```python
from build123d import *

# Parameters (mm, degrees)
SKETCH1_W           = 101.6
SKETCH1_H           = 247.65
BOSS_EXTRUDE1_DEPTH = 152.4
SKETCH2_R           = 15.08125
SKETCH2_R_2         = 9.525
CUT_EXTRUDE1_DEPTH  = 203.827588422
CUT_EXTRUDE2_DEPTH  = 222.090367554
SKETCH33_R          = 2.5796875
CUT_EXTRUDE33_DEPTH = 25.4
SKETCH53_R          = 31.75
CUT_EXTRUDE37_DEPTH = 24.13
SKETCH54_R          = 19.05
CUT_EXTRUDE38_DEPTH = 38.1
SKETCH4_R           = 19.05
CUT_EXTRUDE40_DEPTH = 12.7
SKETCH55_R          = 1.7859375
CUT_EXTRUDE41_DEPTH = 25.4
SKETCH56_R          = 14.2494
CUT_EXTRUDE42_DEPTH = 12.7
CUT_EXTRUDE43_START = -12.7
SKETCH57_R          = 14.2494
CUT_EXTRUDE43_DEPTH = 12.7
SKETCH58_R          = 25.4
CUT_EXTRUDE44_DEPTH = 50.8
CUT_EXTRUDE45_DEPTH = 127
FILLET2_R           = 0.00254
CUT_EXTRUDE46_START = -12.7
SKETCH60_R          = 19.05
CUT_EXTRUDE46_DEPTH = 12.7
SKETCH61_R          = 9.525
CUT_EXTRUDE47_DEPTH = 222.090367554
SKETCH62_R          = 2.0193
CUT_EXTRUDE48_DEPTH = 25.4
SKETCH63_R          = 3.175
CUT_EXTRUDE49_DEPTH = 12.7


with BuildPart() as part:
    # Sketch1 → Boss-Extrude1 (new body)
    with BuildSketch(Plane.XY):
        Rectangle(SKETCH1_W, SKETCH1_H)
    extrude(amount=BOSS_EXTRUDE1_DEPTH)

    # Sketch2 → Cut-Extrude1 (cut, through all)
    with BuildSketch(Plane(origin=(0, 0, 0), x_dir=(-1, 0, 0), z_dir=(0, 0, -1))):
        with Locations((0, -60.579)):
            Circle(SKETCH2_R)
        with Locations((0, 53.721)):
            Circle(SKETCH2_R_2)
    extrude(amount=-CUT_EXTRUDE1_DEPTH, mode=Mode.SUBTRACT)

    # Sketch3 → Cut-Extrude2 (cut, through all)
    with BuildSketch(Plane.ZY.offset(50.8)):
        Polygon((152.4, -60.325), (88.9, -123.825), (152.4, -123.825), align=None)
    extrude(amount=-CUT_EXTRUDE2_DEPTH, mode=Mode.SUBTRACT)

    # Sketch33 → Cut-Extrude33 (cut)
    with BuildSketch(Plane(origin=(0, 0, 0), x_dir=(-1, 0, 0), z_dir=(0, 0, -1))):
        with Locations((-40.005, 102.9335)):
            Circle(SKETCH33_R)
        with Locations((40.005, 102.9335)):
            Circle(SKETCH33_R)
        with Locations((40.005, 4.5085)):
            Circle(SKETCH33_R)
        with Locations((-40.005, 4.5085)):
            Circle(SKETCH33_R)
    extrude(amount=-CUT_EXTRUDE33_DEPTH, mode=Mode.SUBTRACT)

    # Sketch53 → Cut-Extrude37 (cut)
    with BuildSketch(Plane(origin=(0, 0, 0), x_dir=(-1, 0, 0), z_dir=(0, 0, -1))):
        with Locations((0, -60.579)):
            Circle(SKETCH53_R)
    extrude(amount=-CUT_EXTRUDE37_DEPTH, mode=Mode.SUBTRACT)

    # Sketch54 → Cut-Extrude38 (cut)
    with BuildSketch(Plane(origin=(0, 0, 0), x_dir=(-1, 0, 0), z_dir=(0, 0, -1))):
        with Locations((0, 53.721)):
            Circle(SKETCH54_R)
    extrude(amount=-CUT_EXTRUDE38_DEPTH, mode=Mode.SUBTRACT)

    # Sketch4 → Cut-Extrude40 (cut)
    with BuildSketch(Plane(origin=(50.8, 0, 0), x_dir=(0, 0, -1), z_dir=(1, 0, 0))):
        with Locations((-76.2, 28.575)):
            Circle(SKETCH4_R)
    extrude(amount=-CUT_EXTRUDE40_DEPTH, mode=Mode.SUBTRACT)

    # Sketch55 → Cut-Extrude41 (cut)
    with BuildSketch(Plane.ZY.offset(50.8)):
        with Locations((52.3875, 28.575)):
            Circle(SKETCH55_R)
        with Locations((64.29375, 49.197229928)):
            Circle(SKETCH55_R)
        with Locations((88.10625, 49.197229928)):
            Circle(SKETCH55_R)
        with Locations((100.0125, 28.575)):
            Circle(SKETCH55_R)
        with Locations((88.10625, 7.952770072)):
            Circle(SKETCH55_R)
        with Locations((64.29375, 7.952770072)):
            Circle(SKETCH55_R)
    cut_extrude41 = extrude(amount=-CUT_EXTRUDE41_DEPTH, mode=Mode.SUBTRACT)

    # Sketch56 → Cut-Extrude42 (cut)
    with BuildSketch(Plane.XY.offset(152.4)):
        with Locations((0, 53.721)):
            Circle(SKETCH56_R)
    extrude(amount=-CUT_EXTRUDE42_DEPTH, mode=Mode.SUBTRACT)

    # Sketch57 → Cut-Extrude43 (cut)
    with BuildSketch(Plane(origin=(0, 0, 38.1), x_dir=(-1, 0, 0), z_dir=(0, 0, -1)).offset(CUT_EXTRUDE43_START)):
        with Locations(Location((0, 53.721, 0), (0, 0, 180))):
            Circle(SKETCH57_R)
    extrude(amount=CUT_EXTRUDE43_DEPTH, mode=Mode.SUBTRACT)

    # Sketch58 → Cut-Extrude44 (cut)
    with BuildSketch(Plane.XY.offset(152.4)):
        with Locations((0, -60.579)):
            Circle(SKETCH58_R)
    extrude(amount=-CUT_EXTRUDE44_DEPTH, mode=Mode.SUBTRACT)

    # Sketch59 → Cut-Extrude45 (cut)
    with BuildSketch(Plane.XY.offset(152.4)):
        with BuildLine():
            ThreePointArc((-17.734642857, -13.34047826), (20.0025, -4.0894), (-17.734642857, 5.16167826))
            ThreePointArc((-17.734642857, 5.16167826), (-29.5275, -4.0894), (-17.734642857, -13.34047826))
        make_face()
    extrude(amount=-CUT_EXTRUDE45_DEPTH, mode=Mode.SUBTRACT)

    # Fillet2
    fillet2_edges = [part.edges().sort_by_distance(p)[0] for p in [
        (50.8, -123.825, 44.45),
        (-50.8, -123.825, 44.45),
        (-50.8, 123.825, 76.2),
        (50.8, 123.825, 76.2),
    ]]
    fillet(fillet2_edges, radius=FILLET2_R)

    # Sketch60 → Cut-Extrude46 (cut)
    with BuildSketch(Plane.ZY.offset(50.8).offset(CUT_EXTRUDE46_START)):
        with Locations(Location((76.2, 28.575, 0), (0, 0, 180))):
            Circle(SKETCH60_R)
    extrude(amount=CUT_EXTRUDE46_DEPTH, mode=Mode.SUBTRACT)

    # Sketch61 → Cut-Extrude47 (cut, through all)
    with BuildSketch(Plane(origin=(50.8, 0, 0), x_dir=(0, 0, -1), z_dir=(1, 0, 0))):
        with Locations((-76.2, 28.575)):
            Circle(SKETCH61_R)
    extrude(amount=-CUT_EXTRUDE47_DEPTH, mode=Mode.SUBTRACT)

    # Sketch62 → Cut-Extrude48 (cut)
    with BuildSketch(Plane.XY.offset(152.4)):
        with Locations((-22.225, 18.1356)):
            Circle(SKETCH62_R)
        with Locations((22.225, 18.1356)):
            Circle(SKETCH62_R)
        with Locations((22.225, -26.3144)):
            Circle(SKETCH62_R)
        with Locations((-22.225, -26.3144)):
            Circle(SKETCH62_R)
    extrude(amount=-CUT_EXTRUDE48_DEPTH, mode=Mode.SUBTRACT)

    # Sketch63 → Cut-Extrude49 (cut)
    with BuildSketch(Plane(origin=(50.8, 0, 0), x_dir=(0, 0, -1), z_dir=(1, 0, 0))):
        with Locations((-50.8, 66.675)):
            Circle(SKETCH63_R)
        with Locations((-12.7, 66.675)):
            Circle(SKETCH63_R)
        with Locations((-12.7, 92.075)):
            Circle(SKETCH63_R)
        with Locations((-50.8, 92.075)):
            Circle(SKETCH63_R)
    extrude(amount=-CUT_EXTRUDE49_DEPTH, mode=Mode.SUBTRACT)

    # Mirror2: Cut-Extrude41 across plane
    add(cut_extrude41.mirror(Plane(origin=(0, 0, 0), x_dir=(0, 0, 1), z_dir=(1, 0, 0))), mode=Mode.SUBTRACT)


solid = part.part
```
Part model, mm, in its own coordinate system. A direction names the side the tool comes from. Round coordinates to 2 decimals unless told otherwise and drop trailing zeros. Order: outer loops, then holes, each group sorted by start corner. A loop starts at its lowest first (then second) coordinate and runs counter-clockwise, first axis right, second up. Notation, with made-up numbers: M 7.25,27.5 L 66.25,27.5 A20 ccw 66.25,54.5 Z; hole C -3,-15 d7. An arc over 180 degrees is marked long. Answer in a Markdown table with one row per item. Add a question column.
Q1. Mould opens along Z. For faces 1 (the face through (-1, 33, 152.4)), 2 (the face through (1.24, 63.165, 94.628)), 3 (the face through (0.533, 28.994, 85.716)) say: +Z half, -Z half, draft (parallel to the pull), parting line (faces both ways), or undercut.
Q2. Pin check, flat tips, straight feed: pin 1 (1.9 mm diameter, centred on y = 66, z = 51.5, fed in from +X); pin 2 (4 mm diameter, centred on x = -40.01, y = 4.51, fed in from -Z); pin 3 (2 mm diameter, centred on y = 49.2, z = 88.11, fed in from +X). Stop position of each tip, or through.
Q3. Cut at A-A on z = 78. Give the number of separate pieces and of enclosed holes in the cut face, and give its area (3 significant figures).
Q4. Wall check: L1, parallel to Y at x = 0, z = 141 (3 decimals); L2, parallel to Y at x = 0, z = 5 (3 decimals); L3, parallel to X at y = -26.5, z = 133. Give the ranges that are in metal, low to high. Write a range as from..to.
Q5. Cut at C-C on y = -73. Give the cut face in (x, z) (3 decimals).
Q6. 3-axis set-ups, long thin cutter, end or side, ignore diameter. For faces 4 (the face through (3, 63, 50.8)), 5 (the face through (38.1, 92, 13)), 6 (the face through (-38.1, 33, 85)): which of +Z, -Z, +X, -X, +Y, -Y reach the whole face in a straight line?
Established:
| question | item | result |
|---|---|---|
| 1 | face 1 | +Z half |
| 1 | face 2 | draft |
| 1 | face 3 | undercut |
| 2 | pin 1 | stops at x = 38.1 |
| 2 | pin 2 | stops at z = 25.4 |
| 2 | pin 3 | stops at x = 25.4 |
| 3 | separate pieces | 2 |
| 3 | enclosed holes | 3 |
| 3 | area | 20,400 mm2 |
| 4 | L1 | y = -35.179..-24.092, 15.913..39.472, 67.97..123.825 |
| 4 | L2 | y = -123.825..-92.329, -28.829..34.671, 72.771..123.825 |
| 4 | L3 | x = -50.8..-24.24, -20.21..20.21, 24.24..50.8 |
| 5 | outline | M -50.8,0 L -29.22,0 L -29.22,24.13 L -8.554,24.13 L -8.554,101.6 L -22.156,101.6 L -22.156,139.725 L -50.8,139.725 Z; M 8.554,24.13 L 29.22,24.13 L 29.22,0 L 50.8,0 L 50.8,139.725 L 22.156,139.725 L 22.156,101.6 L 8.554,101.6 Z |
| 6 | face 4 | -Z |
| 6 | face 5 | +X |
| 6 | face 6 | -X |
